```python
from build123d import *

# Parameters (mm, degrees)
ESBO_O1_W                  = 90.2
ESBO_O1_H                  = 95.9
RESSALTO_EXTRUS_O1_DEPTH   = 3.5
ESBO_O2_R                  = 1.25
CORTE_EXTRUS_O1_DEPTH      = 5
CORTE_EXTRUS_O3_DEPTH      = 5
ESBO_O4_R                  = 1.25
CORTE_EXTRUS_O2_DEPTH      = 10
CHANFRO4_SIZE              = 1.75
CHANFRO5_SIZE              = 1.75
CHANFRO6_SIZE              = 2.25
CHANFRO7_SIZE              = 2.25
CORTE_EXTRUS_O4_DEPTH      = 0.2
CORTE_EXTRUS_O5_DEPTH      = 0.2
CORTE_EXTRUS_O7_DEPTH      = 66.920122118
CORTE_EXTRUS_O7_DEPTH_BACK = 5
ESBO_O7_W                  = 1.6
ESBO_O7_H                  = 6.5
CORTE_EXTRUS_O8_DEPTH      = 5
ESBO_O9_W                  = 1.346153846
ESBO_O9_H                  = 0.358974359
CORTE_EXTRUS_O9_DEPTH      = 0.2


with BuildPart() as part:
    # Esboço1 → Ressalto-extrusão1 (new body)
    with BuildSketch(Plane.XY):
        Rectangle(ESBO_O1_W, ESBO_O1_H)
    extrude(amount=RESSALTO_EXTRUS_O1_DEPTH)

    # Esboço2 → Corte-extrusão1 (cut)
    with BuildSketch(Plane.XY):
        with Locations((-36.2, 42.85)):
            Circle(ESBO_O2_R)
        with Locations((37.5, 42.85)):
            Circle(ESBO_O2_R)
        with Locations((40, -42.85)):
            Circle(ESBO_O2_R)
        with Locations((-40, -42.85)):
            Circle(ESBO_O2_R)
    extrude(amount=CORTE_EXTRUS_O1_DEPTH, mode=Mode.SUBTRACT)

    # Esboço3 → Corte-extrusão3 (cut)
    with BuildSketch(Plane.XY):
        Polygon((-26.25, 41.25), (26.25, 41.25), (41.25, 26.25), (41.25, -26.25), (26.25, -41.25), (-26.25, -41.25), (-41.25, -26.25), (-41.25, 26.25), align=None)
    extrude(amount=CORTE_EXTRUS_O3_DEPTH, mode=Mode.SUBTRACT)

    # Esboço4 → Corte-extrusão2 (cut)
    with BuildSketch(Plane.XY):
        with Locations((-36.25, 36.25)):
            Circle(ESBO_O4_R)
        with Locations((36.25, 36.25)):
            Circle(ESBO_O4_R)
        with Locations((-36.25, -36.25)):
            Circle(ESBO_O4_R)
        with Locations((36.25, -36.25)):
            Circle(ESBO_O4_R)
    extrude(amount=CORTE_EXTRUS_O2_DEPTH, mode=Mode.SUBTRACT)

    # Chanfro4
    chanfro4_edges = [part.edges().sort_by_distance(p)[0] for p in [
        (-41.25, -42.85, 3.5),
    ]]
    chamfer(chanfro4_edges, length=CHANFRO4_SIZE)

    # Chanfro5
    chanfro5_edges = [part.edges().sort_by_distance(p)[0] for p in [
        (38.75, -42.85, 3.5),
    ]]
    chamfer(chanfro5_edges, length=CHANFRO5_SIZE)

    # Chanfro6
    chanfro6_edges = [part.edges().sort_by_distance(p)[0] for p in [
        (-37.45, 42.85, 3.5),
    ]]
    chamfer(chanfro6_edges, length=CHANFRO6_SIZE)

    # Chanfro7
    chanfro7_edges = [part.edges().sort_by_distance(p)[0] for p in [
        (36.25, 42.85, 3.5),
    ]]
    chamfer(chanfro7_edges, length=CHANFRO7_SIZE)

    # Esboço5 → Corte-extrusão4 (cut)
    with BuildSketch(Plane.XY.offset(3.5)):
        Polygon((-34.011664728, -41.359633286), (-33.364529311, -41.359633286), (-33.364529311, -44.859633286), (-33.678631875, -44.859633286), (-33.678631875, -41.718607645), (-34.217093414, -41.718607645), align=None)
    extrude(amount=-CORTE_EXTRUS_O4_DEPTH, mode=Mode.SUBTRACT)

    # Esboço6 → Corte-extrusão5 (cut)
    with BuildSketch(Plane(origin=(0, 0, 0), x_dir=(-1, 0, 0), z_dir=(0, 0, -1))):
        Polygon((33.93825461, -40.504659527), (34.585390027, -40.504659527), (34.585390027, -44.004659527), (34.271287463, -44.004659527), (34.271287463, -40.863633886), (33.732825924, -40.863633886), align=None)
    extrude(amount=-CORTE_EXTRUS_O5_DEPTH, mode=Mode.SUBTRACT)

    # Esboço7 → Corte-extrusão7 (cut, two sides: drawn at the far end of the back side and taken through both)
    with BuildSketch(Plane(origin=(0, 0, 0), x_dir=(-1, 0, 0), z_dir=(0, 0, -1)).offset(-CORTE_EXTRUS_O7_DEPTH_BACK)):
        with Locations((-44.3, -44.7)):
            Rectangle(ESBO_O7_W, ESBO_O7_H)
    extrude(amount=CORTE_EXTRUS_O7_DEPTH + CORTE_EXTRUS_O7_DEPTH_BACK, mode=Mode.SUBTRACT)

    # Esboço8 → Corte-extrusão8 (cut)
    with BuildSketch(Plane.XY.offset(3.5)):
        Polygon((-43.5, 47.95), (-43.5, 41.45), (-45.1, 41.45), (-45.287231685, 41.45), (-45.287231685, 48.410891955), (-43.5, 48.410891955), align=None)
    extrude(amount=-CORTE_EXTRUS_O8_DEPTH, mode=Mode.SUBTRACT)

    # Esboço9 → Corte-extrusão9 (cut)
    with BuildSketch(Plane.XY.offset(3.5)):
        with Locations((-1.407956652, -44.741681875)):
            Rectangle(ESBO_O9_W, ESBO_O9_H)
        Polygon((-0.46564896, -43.530143413), (1.46383822, -43.530143413), (-0.023942229, -45.773733157), (1.418966425, -45.773733157), (1.418966425, -46.087835721), (-0.600264345, -46.087835721), (0.888217226, -43.844245977), (-0.46564896, -43.844245977), align=None)
    extrude(amount=-CORTE_EXTRUS_O9_DEPTH, mode=Mode.SUBTRACT)


solid = part.part
```
Can you work these out from the model? Positions are in its coordinate system, mm. A direction names the side the tool comes from. Round coordinates to 2 decimals unless told otherwise and drop trailing zeros. Loops run counter-clockwise (first coordinate to the right, second up) from the corner with the lowest first, then second, coordinate; pieces in that order, holes last. Notation, with made-up numbers: M 37,8.25 L 77,8.25 A14 ccw 77,33.25 Z; hole C 44,37 d3. An arc over 180 degrees is marked long. Answer in a Markdown table with one row per item.
1. If we section it at C-C, the plane x = 8: Please give me the cut outline in (y, z).
Established:
| item | result |
|---|---|
| outline | M -47.95,0 L -41.25,0 L -41.25,3.5 L -47.95,3.5 Z; M 41.25,0 L 47.95,0 L 47.95,3.5 L 41.25,3.5 Z |
2. Please list where these lines run through material, in increasing order: line 1 (X direction, y = 42.85, z = 0.65); line 2 (Y direction, x = -11.5, z = 0.45); line 3 (X direction, y = 17, z = 2.8). Write a range as from..to.
Established:
| item | result |
|---|---|
| line 1 | -43.5..-37.45, -34.95..36.25, 38.75..45.1 |
| line 2 | -47.95..-41.25, 41.25..47.95 |
| line 3 | -45.1..-41.25, 41.25..45.1 |
3. If we section it at B-B, the plane y = 42.85: Please give me the cut outline in (x, z).
Established:
| item | result |
|---|---|
| outline | M -43.5,0 L -37.45,0 L -37.45,1.25 L -39.7,3.5 L -43.5,3.5 Z; M -34.95,0 L 36.25,0 L 36.25,1.25 L 34,3.5 L -32.7,3.5 L -34.95,1.25 Z; M 38.75,0 L 45.1,0 L 45.1,3.5 L 41,3.5 L 38.75,1.25 Z |
4. If we section it at D-D, the plane z = 2.6: Give the number of separate pieces and of enclosed holes in the cut face, plus the area to 3 significant figures.
Established:
| item | result |
|---|---|
| separate pieces | 1 |
| enclosed holes | 9 |
| area | 2,180 mm² |
5. Thinking about a two-plate mould opening in X: for faces 4 (the face through (45.1, 3, 2)), 5 (the face through (39.84, -41.61, 0.86)), 6 (the face through (-45.1, -4, 2)), which applies, pulls with the +X half, pulls with the -X half, needs draft (parallel to the pull), parting line crosses it, or undercut?
Established:
| item | result |
|---|---|
| face 4 | pulls with the +X half |
| face 5 | undercut |
| face 6 | pulls with the -X half |
6. On a 3-axis mill with a long thin cutter (end or side, diameter ignored), from which of +Z, -Z, +X, -X, +Y, -Y can I reach the whole of each face in a straight line? I mean faces 1 (the face through (43.5, -45, 2)), 2 (the face through (38.756, 43.371, 1.359)), 3 (the face through (-33.6, -33.9, 1.7)). Say none if no direction works.
Established:
| item | result |
|---|---|
| face 1 | +Z, -Z, +X, -Y |
| face 2 | +Z |
| face 3 | +Z, -Z |
7. I'm going to push flat-ended pins straight in: pin 1 Ø0.8 at (x, z) = (-44, 2) entering from +Y; pin 2 Ø10 at (x, y) = (-20, 34.5) entering from -Z. Where does each tip first touch, or does it pass through?
Established:
| item | result |
|---|---|
| pin 1 | y = 41.45 |
| pin 2 | through |
8. If we section it at A-A, the plane y = -23.5: Please give me the cut outline in (x, z), plus the area to 4 significant figures.
Established:
| item | result |
|---|---|
| outline | M -45.1,0 L -41.25,0 L -41.25,3.5 L -45.1,3.5 Z; M 41.25,0 L 45.1,0 L 45.1,3.5 L 41.25,3.5 Z |
| area | 26.95 mm² |
